Here's how the part is built. I have some questions about the finished solid (model axes, mm). Face numbers are marked on the shaded views. Coordinates: 2 decimals unless noted, no trailing zeros. Write each loop counter-clockwise with the first axis right and the second up, starting at its lowest first coordinate (ties: lowest second). Pieces come first, ordered by that corner, then holes. Notation, with made-up numbers: M -33.5,88 L -18.5,88 A7 ccw -18.5,97 Z; hole C 14.25,73.5 d9. An arc over 180 degrees is marked long. Use a Markdown table: item, result.
```python
from build123d import *

# Parameters (mm, degrees)
SKETCH1_W           = 70
SKETCH1_H           = 26
BOSS_EXTRUDE1_DEPTH = 5
SHELL1_T            = -1.5
SKETCH2_R           = 0.75
CUT_EXTRUDE1_DEPTH  = 2.5


with BuildPart() as part:
    # Sketch1 → Boss-Extrude1 (new body)
    with BuildSketch(Plane.XY):
        Rectangle(SKETCH1_W, SKETCH1_H)
    extrude(amount=BOSS_EXTRUDE1_DEPTH)

    # Shell1
    shell1_openings = [part.faces().sort_by_distance(p)[0] for p in [
        (0, 0, 5),
    ]]
    offset(amount=SHELL1_T, openings=shell1_openings, kind=Kind.INTERSECTION)

    # Sketch2 → Cut-Extrude1 (cut, through all)
    with BuildSketch(Plane.XY.offset(1.5)):
        with Locations((-21.5, 0)):
            Circle(SKETCH2_R)
        with Locations((3.5, 0)):
            Circle(SKETCH2_R)
    extrude(amount=-CUT_EXTRUDE1_DEPTH, mode=Mode.SUBTRACT)


solid = part.part
```
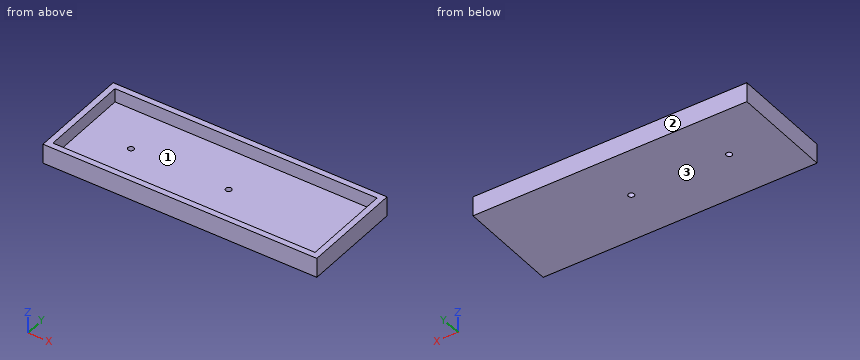
1. Suppose I cut it at B-B on x = 3.5. Write out the boundary of the cut face in (y, z).
Answers follow:
| item | result |
|---|---|
| outline | M -13,0 L -0.75,0 L -0.75,1.5 L -11.5,1.5 L -11.5,5 L -13,5 Z; M 0.75,0 L 13,0 L 13,5 L 11.5,5 L 11.5,1.5 L 0.75,1.5 Z |
2. I need wall thicknesses on probe 1 along Y at (x, z) = (2.5, 3.3); probe 2 along Y at (x, z) = (3.5, 1.15); probe 3 along X at (y, z) = (4.5, 2.75). Which ranges of each line are inside material? Lowest first, please.
Answers follow:
| item | result |
|---|---|
| probe 1 | y = -13 to -11.5, 11.5 to 13 |
| probe 2 | y = -13 to -0.75, 0.75 to 13 |
| probe 3 | x = -35 to -33.5, 33.5 to 35 |
3. Suppose I cut it at D-D on x = -27. Write out the boundary of the cut face in (y, z).
Answers follow:
| item | result |
|---|---|
| outline | M -13,0 L 13,0 L 13,5 L 11.5,5 L 11.5,1.5 L -11.5,1.5 L -11.5,5 L -13,5 Z |
4. Suppose I cut it at C-C on z = 3. Write out the boundary of the cut face in (x, y).
Answers follow:
| item | result |
|---|---|
| outline | M -35,-13 L 35,-13 L 35,13 L -35,13 Z; hole M -33.5,-11.5 L 33.5,-11.5 L 33.5,11.5 L -33.5,11.5 Z |
5. We'd pull the mould along Y, two halves only. Please class the marked faces 1, 2 and 3: +Y half, -Y half, draft (parallel to the pull), parting line (faces both ways), or undercut.
Answers follow:
| item | result |
|---|---|
| face 1 | undercut |
| face 2 | +Y half |
| face 3 | draft |
6. Will these pins go through, and if not, where does the flat tip stop? pin 1 Ø2 at (x, y) = (-21.5, 0) entering from -Z; pin 2 Ø8 at (x, y) = (-17.5, -4) entering from +Z; pin 3 Ø1.2 at (x, y) = (3.5, 0) entering from +Z.
Answers follow:
| item | result |
|---|---|
| pin 1 | stops at z = 0 |
| pin 2 | stops at z = 1.5 |
| pin 3 | passes through |
7. Suppose I cut it at A-A on y = 0. Write out the boundary of the cut face in (x, z), and give its area (3 significant figures).
Answers follow:
| item | result |
|---|---|
| outline | M -35,0 L -22.25,0 L -22.25,1.5 L -33.5,1.5 L -33.5,5 L -35,5 Z; M -20.75,0 L 2.75,0 L 2.75,1.5 L -20.75,1.5 Z; M 4.25,0 L 35,0 L 35,5 L 33.5,5 L 33.5,1.5 L 4.25,1.5 Z |
| area | 111 mm2 |
